Study the drawing (mm; zero at the part's minimum x, y, z) and answer. A direction names the side the tool comes from. Give positions to 0.01 mm unless a question says otherwise; leave off trailing zeros. Order: outer loops, then holes, each group sorted by start corner. A loop starts at its lowest first (then second) coordinate and runs counter-clockwise, first axis right, second up. Notation, with made-up numbers: (23.25, 76) -> (78.25, 76) arc R24 cw to (78.25, 101) -> close; hole circle Ø1 at (-3, 4.5). An arc over 180 degrees is marked (long way). Use a Markdown table: item, result. Add a question column.
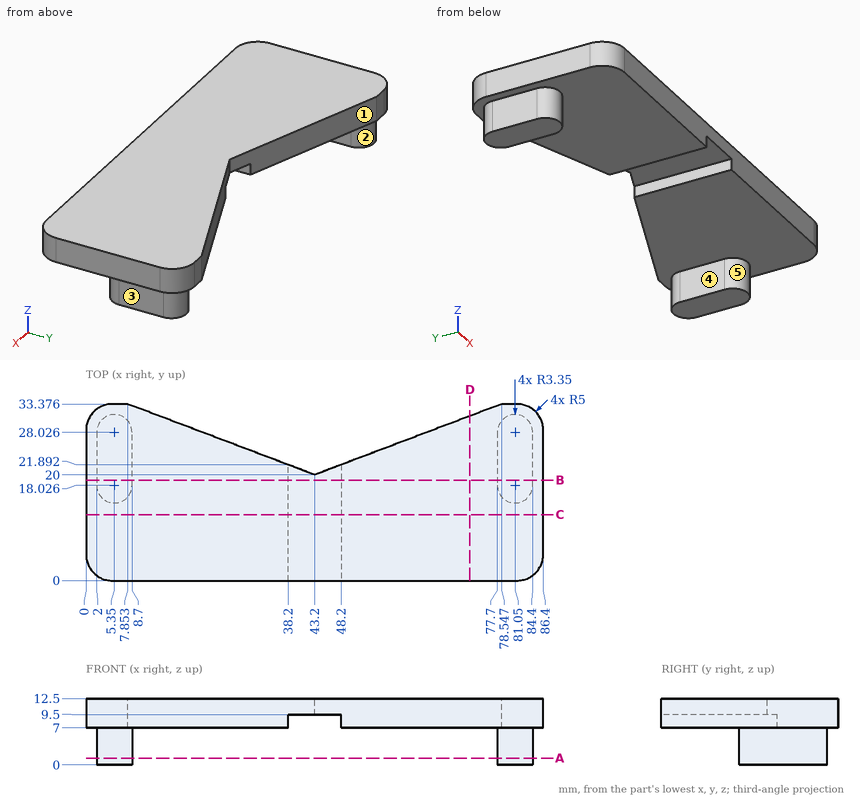
1) Which of the six approach directions +Z, -Z, +X, -X, +Y, -Y give full straight-line access (tool end or side, diameter ignored) to the marked faces 1, 2, 3, 4 and 5?
2) The part is cut by section B-B, the plane y = 19. Determine the outline of the cut face in (x, z), then the cut area to 3 significant figures.
3) The part is cut by section A-A, the plane z = 1.25. Determine the outline of the cut face in (x, y).
4) The part is cut by section C-C, the plane y = 12.5. Determine the outline of the cut face in (x, z).
5) Straight lines are drawn through the part: line 1 (X direction, y = 21, z = 6); line 2 (X direction, y = 19, z = 8.25); line 3 (Z direction, x = 33, y = 18). For each, find the intervals that lie inside material, in ascending order.
6) Flat-ended cylindrical pins translate along their axes: pin 1 (16.5 mm diameter, centred on x = 25.5, y = 24, fed in from -Z); pin 2 (5 mm diameter, centred on y = 29.5, z = 2, fed in from +X); pin 3 (5.5 mm diameter, centred on y = 25, z = 3.5, fed in from -X). Find the tip coordinate at first contact, or state that the pin passes through.
7) The part is cut by section D-D, the plane x = 72.5. Determine the outline of the cut face in (y, z).
A:
| question | item | result |
|---|---|---|
| 1 | face 1 | +Z, -Z, +Y |
| 1 | face 2 | -Z, +Y |
| 1 | face 3 | -Z, +X, +Y, -Y |
| 1 | face 4 | -Z, +Y, -Y |
| 1 | face 5 | -Z, -Y |
| 2 | outline | (0, 7) -> (2, 7) -> (2, 0) -> (8.7, 0) -> (8.7, 7) -> (38.2, 7) -> (38.2, 9.5) -> (48.2, 9.5) -> (48.2, 7) -> (77.7, 7) -> (77.7, 0) -> (84.4, 0) -> (84.4, 7) -> (86.4, 7) -> (86.4, 12.5) -> (0, 12.5) -> close |
| 2 | area | 544 mm^2 |
| 3 | outline | (2, 18.03) arc R3.35 ccw to (8.7, 18.03) -> (8.7, 28.03) arc R3.35 ccw to (2, 28.03) -> close; (77.7, 18.03) arc R3.35 ccw to (84.4, 18.03) -> (84.4, 28.03) arc R3.35 ccw to (77.7, 28.03) -> close |
| 4 | outline | (0, 7) -> (38.2, 7) -> (38.2, 9.5) -> (48.2, 9.5) -> (48.2, 7) -> (86.4, 7) -> (86.4, 12.5) -> (0, 12.5) -> close |
| 5 | line 1 | 2 to 8.7, 77.7 to 84.4 |
| 5 | line 2 | 0 to 38.2, 48.2 to 86.4 |
| 5 | line 3 | 7 to 12.5 |
| 6 | pin 1 | z = 7 |
| 6 | pin 2 | x = 84.4 |
| 6 | pin 3 | x = 2 |
| 7 | outline | (0, 7) -> (31.09, 7) -> (31.09, 12.5) -> (0, 12.5) -> close |
